Source: CAD feature listing. Evaluate the final solid. Frame: model axes, mm. Face numbers are marked on the shaded views. A direction names the side the tool comes from. Give positions to 0.01 mm unless a question says otherwise; leave off trailing zeros. Order: outer loops, then holes, each group sorted by start corner. A loop starts at its lowest first (then second) coordinate and runs counter-clockwise, first axis right, second up. Notation, with made-up numbers: M 35.5,42.5 L 63.5,42.5 A5 cw 63.5,50.5 Z; hole C -18,-4.5 d11. An arc over 180 degrees is marked long. Answer as a JSON object with one key per item and string values. Group by question number.
1. Material intervals for L1, parallel to Y at x = 13, z = 5.25; L2, parallel to X at y = 5, z = 1.7 (3 decimals); L3, parallel to Z at x = -3.5, y = 8.5, sorted ascending. Write a range as [from, to].
2. Set-up query: the marked faces 1, 2, 3 and 4. Return all of +Z, -Z, +X, -X, +Y, -Y with unobstructed straight access to the full face (end or side cutting, diameter ignored); none if empty.
3. Section query B-B (y = 0). Output: boundary loops of the cut face in (x, z) (3 decimals).
4. Pull-direction query (Y, two-part tool) for the marked faces 5, 6 and 7; classes: +Y half, -Y half, draft (parallel to the pull), parting line (faces both ways), or undercut.
5. Section query C-C (z = 4). Output: boundary loops of the cut face in (x, y), plus the area to 3 significant figures.
6. Pin query (flat end, axial travel): P1, Ø1.1, axis at x = 0.5, y = 1, coming from the -Z side; P2, Ø10, axis at x = 2.5, y = 8, coming from the -Z side; P3, Ø3, axis at x = 2, z = 4, coming from the +Y side. Return the tip coordinate at first contact, or that it passes through.
7. Section query A-A (x = -10.5). Output: boundary loops of the cut face in (y, z), plus the area to 3 significant figures.
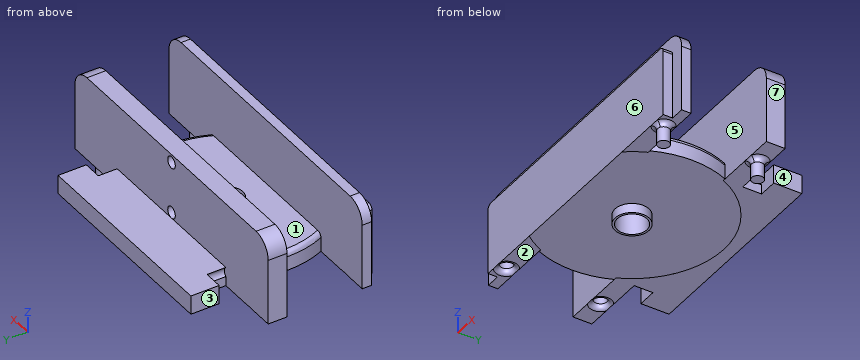
from build123d import *

# Parameters (mm, degrees)
BOSS_EXTRUDE1_DEPTH     = 2
SKETCH2_R               = 1.575
BOSS_EXTRUDE2_DEPTH     = 4
SKETCH3_R               = 1.8
BOSS_EXTRUDE3_DEPTH     = 1
SKETCH4_W               = 2
SKETCH4_H               = 17
BOSS_EXTRUDE4_DEPTH     = 0.001
SKETCH5_W               = 18
SKETCH5_H               = 2
BOSS_EXTRUDE5_DEPTH     = 0.001
SKETCH6_W               = 2.001
SKETCH6_H               = 2
BOSS_EXTRUDE6_DEPTH     = 5
BOSS_EXTRUDE7_DEPTH     = 0.001
CUT_EXTRUDE1_DEPTH      = 20.519323784
SKETCH9_W               = 2.937742252
SKETCH9_H               = 8
CUT_EXTRUDE2_DEPTH      = 0.001
CUT_EXTRUDE11_START     = -0.001
SKETCH21_R              = 9.75
SKETCH21_R_2            = 1.8
CUT_EXTRUDE11_DEPTH     = 0.001
SKETCH10_W              = 32
SKETCH10_H              = 2
BOSS_EXTRUDE8_DEPTH     = 7
FILLET1_R               = 0.5
SKETCH11_R              = 0.625
BOSS_EXTRUDE9_DEPTH     = 2
SKETCH14_W              = 2
SKETCH14_H              = 2
CUT_EXTRUDE5_DEPTH      = 22.401355237
SKETCH12_R              = 0.675
CUT_EXTRUDE3_DEPTH      = 2.5
CUT_EXTRUDE6_DEPTH      = 2
FILLET2_R               = 0.5
FILLET3_R               = 0.5
FILLET4_R               = 2
CUT_EXTRUDE7_DEPTH      = 26.019992106
CUT_EXTRUDE7_DEPTH_BACK = 1
SKETCH19_R              = 0.625
CUT_EXTRUDE9_DEPTH      = 2


with BuildPart() as part:
    # Sketch1 → Boss-Extrude1 (new body)
    with BuildSketch(Plane.XY):
        Polygon((-11, 6), (-11, 11), (11, 11), (11, 6), (11, -6), (-11, -6), align=None)
    extrude(amount=BOSS_EXTRUDE1_DEPTH)

    # Sketch3 → Boss-Extrude3 (add)
    with BuildSketch(Plane(origin=(0, 0, 0), x_dir=(-1, 0, 0), z_dir=(0, 0, -1))):
        with Locations(Location((0, 0, 0), (0, 0, 180))):
            Circle(SKETCH3_R)
    extrude(amount=BOSS_EXTRUDE3_DEPTH)

    # Sketch4 → Boss-Extrude4 (add)
    with BuildSketch(Plane(origin=(0, 0, 0), x_dir=(-1, 0, 0), z_dir=(0, 0, -1))):
        with Locations((10, 2.5)):
            Rectangle(SKETCH4_W, SKETCH4_H)
        with Locations((-10, 2.5)):
            Rectangle(SKETCH4_W, SKETCH4_H)
    extrude(amount=BOSS_EXTRUDE4_DEPTH)

    # Sketch5 → Boss-Extrude5 (add)
    with BuildSketch(Plane(origin=(0, 0, 0), x_dir=(-1, 0, 0), z_dir=(0, 0, -1))):
        with Locations((0, 10)):
            Rectangle(SKETCH5_W, SKETCH5_H)
    extrude(amount=BOSS_EXTRUDE5_DEPTH)

    # Sketch6 → Boss-Extrude6 (add)
    with BuildSketch(Plane(origin=(11, 0, 0), x_dir=(0, 0, -1), z_dir=(1, 0, 0))):
        with Locations((-0.9995, -5)):
            Rectangle(SKETCH6_W, SKETCH6_H)
        with Locations((-0.9995, 5)):
            Rectangle(SKETCH6_W, SKETCH6_H)
    boss_extrude6 = extrude(amount=BOSS_EXTRUDE6_DEPTH)

    # Mirror1: Boss-Extrude6 across plane
    add(boss_extrude6.mirror(Plane(origin=(0, 0, 0), x_dir=(0, 0, 1), z_dir=(1, 0, 0))))

    # Sketch7 → Boss-Extrude7 (add)
    with BuildSketch(Plane(origin=(0, 0, -0.001), x_dir=(-1, 0, 0), z_dir=(0, 0, -1))):
        with BuildLine():
            ThreePointArc((-6.708203932, -6), (-8.407551231, -3.211398808), (-9, 0))
            Line((-9, 0), (-9, -6))
            Line((-9, -6), (-6.708203932, -6))
        make_face()
        with BuildLine():
            Line((-9, 9), (-9, 0))
            ThreePointArc((-9, 0), (-6.363961031, 6.363961031), (0, 9))
            Line((0, 9), (-9, 9))
        make_face()
    boss_extrude7 = extrude(amount=-BOSS_EXTRUDE7_DEPTH)

    # Sketch8 → Cut-Extrude1 (cut, through all)
    with BuildSketch(Plane(origin=(0, 0, -0.001), x_dir=(-1, 0, 0), z_dir=(0, 0, -1))):
        with BuildLine():
            Line((-11, 4), (-9.16515139, 4))
            ThreePointArc((-9.16515139, 4), (-10, 0), (-9.16515139, -4))
            Line((-9.16515139, -4), (-11, -4))
            Line((-11, -4), (-11, 4))
        make_face()
    cut_extrude1 = extrude(amount=-CUT_EXTRUDE1_DEPTH, mode=Mode.SUBTRACT)

    # Sketch9 → Cut-Extrude2 (cut)
    with BuildSketch(Plane(origin=(0, 0, -0.001), x_dir=(-1, 0, 0), z_dir=(0, 0, -1))):
        with Locations((-9.531128874, 0)):
            Rectangle(SKETCH9_W, SKETCH9_H)
    cut_extrude2 = extrude(amount=-CUT_EXTRUDE2_DEPTH, mode=Mode.SUBTRACT)

    # Mirror2: Boss-Extrude7, Cut-Extrude1, Cut-Extrude2 across plane
    add(boss_extrude7.mirror(Plane(origin=(0, 0, 0), x_dir=(0, 0, 1), z_dir=(1, 0, 0))))
    add(cut_extrude1.mirror(Plane(origin=(0, 0, 0), x_dir=(0, 0, 1), z_dir=(1, 0, 0))), mode=Mode.SUBTRACT)
    add(cut_extrude2.mirror(Plane(origin=(0, 0, 0), x_dir=(0, 0, 1), z_dir=(1, 0, 0))), mode=Mode.SUBTRACT)

    # Sketch21 → Cut-Extrude11 (cut)
    with BuildSketch(Plane(origin=(0, 0, -0.001), x_dir=(-1, 0, 0), z_dir=(0, 0, -1)).offset(CUT_EXTRUDE11_START)):
        Circle(SKETCH21_R)
        with Locations(Location((0, 0, 0), (0, 0, 180))):
            Circle(SKETCH21_R_2, mode=Mode.SUBTRACT)
    extrude(amount=CUT_EXTRUDE11_DEPTH, mode=Mode.SUBTRACT)

    # Sketch10 → Boss-Extrude8 (add)
    with BuildSketch(Plane.XY.offset(2)):
        with Locations((0, -5)):
            Rectangle(SKETCH10_W, SKETCH10_H)
        with Locations((0, 5)):
            Rectangle(SKETCH10_W, SKETCH10_H)
    extrude(amount=BOSS_EXTRUDE8_DEPTH)

    # Fillet1
    fillet1_edges = [part.edges().sort_by_distance(p)[0] for p in [
        (10, 0, 2),
        (-10, 0, 2),
    ]]
    fillet(fillet1_edges, radius=FILLET1_R)

    # Sketch11 → Boss-Extrude9 (add)
    with BuildSketch(Plane(origin=(0, 0, -0.001), x_dir=(-1, 0, 0), z_dir=(0, 0, -1))):
        with Locations(Location((-13, -5, 0), (0, 0, 180))):
            Circle(SKETCH11_R)
    boss_extrude9 = extrude(amount=BOSS_EXTRUDE9_DEPTH)

    # Sketch14 → Cut-Extrude5 (cut, through all)
    with BuildSketch(Plane(origin=(0, 0, -0.001), x_dir=(-1, 0, 0), z_dir=(0, 0, -1))):
        with Locations((10, 7)):
            Rectangle(SKETCH14_W, SKETCH14_H)
        with Locations((-10, 7)):
            Rectangle(SKETCH14_W, SKETCH14_H)
    extrude(amount=-CUT_EXTRUDE5_DEPTH, mode=Mode.SUBTRACT)

    # Sketch12 → Cut-Extrude3 (cut)
    with BuildSketch(Plane(origin=(0, 0, -0.001), x_dir=(-1, 0, 0), z_dir=(0, 0, -1))):
        with Locations((13, -5)):
            Circle(SKETCH12_R)
    cut_extrude3 = extrude(amount=-CUT_EXTRUDE3_DEPTH, mode=Mode.SUBTRACT)

    # Sketch16 → Cut-Extrude6 (cut)
    with BuildSketch(Plane(origin=(0, 6, 0), x_dir=(1, 0, 0), z_dir=(0, 1, 0))):
        with BuildLine():
            Line((-9, -1), (-9, -2))
            ThreePointArc((-9, -2), (-8.75, -1.5), (-9, -1))
        make_face()
    cut_extrude6 = extrude(amount=CUT_EXTRUDE6_DEPTH, mode=Mode.SUBTRACT)

    # Mirror3: Boss-Extrude9, Cut-Extrude3 across plane
    add(boss_extrude9.mirror(Plane.ZX))
    add(cut_extrude3.mirror(Plane.ZX), mode=Mode.SUBTRACT)

    # Mirror4: Cut-Extrude6 across plane
    add(cut_extrude6.mirror(Plane(origin=(0, 0, 0), x_dir=(0, 0, 1), z_dir=(1, 0, 0))), mode=Mode.SUBTRACT)

    # Fillet2
    fillet2_edges = [part.edges().sort_by_distance(p)[0] for p in [
        (12.375, -5, -0.001),
        (12.375, 5, -0.001),
    ]]
    fillet(fillet2_edges, radius=FILLET2_R)

    # Fillet3
    # the kernel refuses this fillet: 0.5 mm, written as the material it takes off along each edge
    with BuildSketch(Plane(origin=(-13, -5, -0.001), x_dir=(-1, 0, 0), z_dir=(0, -1, 0))) as fillet3_piece_1:
        with BuildLine():
            CenterArc((0.675 + FILLET3_R, -FILLET3_R), FILLET3_R, 90, 90)
            Line((0.675, -FILLET3_R), (0.675, 0))
            Line((0.675, 0), (0.675 + FILLET3_R, 0))
        make_face()
    revolve(axis=Axis((-13, -5, -0.001), (0, 0, -1)), mode=Mode.SUBTRACT)
    with BuildSketch(Plane(origin=(-13, 5, -0.001), x_dir=(-1, 0, 0), z_dir=(0, 1, 0))) as fillet3_piece_2:
        with BuildLine():
            CenterArc((0.675 + FILLET3_R, FILLET3_R), FILLET3_R, 180, 90)
            Line((0.675, FILLET3_R), (0.675, 0))
            Line((0.675, 0), (0.675 + FILLET3_R, 0))
        make_face()
    revolve(axis=Axis((-13, 5, -0.001), (0, 0, 1)), mode=Mode.SUBTRACT)

    # Fillet4
    fillet4_edges = [part.edges().sort_by_distance(p)[0] for p in [
        (16, -5, 9),
        (-16, -5, 9),
        (-16, 5, 9),
        (16, 5, 9),
    ]]
    fillet(fillet4_edges, radius=FILLET4_R)

    # Sketch17 → Cut-Extrude7 (cut, two sides: drawn at the far end of the back side and taken through both)
    with BuildSketch(Plane.XZ.offset(6).offset(-CUT_EXTRUDE7_DEPTH_BACK)):
        with BuildLine():
            Line((-16, 7), (-16, -0.001))
            Line((-16, -0.001), (-14.5, -0.001))
            Line((-14.5, -0.001), (-14.5, 7))
            ThreePointArc((-14.5, 7), (-14.353553391, 7.353553391), (-14, 7.5))
            Line((-14, 7.5), (14, 7.5))
            ThreePointArc((14, 7.5), (14.353553391, 7.353553391), (14.5, 7))
            Line((14.5, 7), (14.5, -0.001))
            Line((14.5, -0.001), (16, -0.001))
            Line((16, -0.001), (16, 7))
            ThreePointArc((16, 7), (15.414213562, 8.414213562), (14, 9))
            Line((14, 9), (-14, 9))
            ThreePointArc((-14, 9), (-15.414213562, 8.414213562), (-16, 7))
        make_face()
    extrude(amount=CUT_EXTRUDE7_DEPTH + CUT_EXTRUDE7_DEPTH_BACK, mode=Mode.SUBTRACT)

    # Sketch19 → Cut-Extrude9 (cut)
    with BuildSketch(Plane(origin=(0, 6, 0), x_dir=(1, 0, 0), z_dir=(0, 1, 0))):
        with Locations(Location((0, -2.625, 0), (0, 0, 90))):
            Circle(SKETCH19_R)
        with Locations(Location((0, -8.125, 0), (0, 0, 270))):
            Circle(SKETCH19_R)
    extrude(amount=-CUT_EXTRUDE9_DEPTH, mode=Mode.SUBTRACT)


with BuildPart() as body_2:
    # Sketch2 → Boss-Extrude2 (new body)
    with BuildSketch(Plane(origin=(0, 0, 2), x_dir=(-1, 0, 0), z_dir=(0, 0, -1))):
        Circle(SKETCH2_R)
    extrude(amount=BOSS_EXTRUDE2_DEPTH)


with BuildPart() as part_1:
    add(part.part)

    # Combine2: cut body 2
    add(body_2.part, mode=Mode.SUBTRACT)


solid = part_1.part
Answer sheet:
{
 "1": {"L1": "[-6, -4], [4, 6]", "L2": "[-16, -13.675], [-12.325, 16]", "L3": "[0, 2]"},
 "2": {"face 1": "+Z, +X, -X", "face 2": "-Z, -X, +Y, -Y", "face 3": "+Z, -Z, -X, +Y", "face 4": "+Z, -Z, +X, +Y"},
 "3": {"outline": "M -10,0 L -1.8,0 L -1.8,-1 L -1.575,-1 L -1.575,2 L -9.5,2 A0.5 ccw -10,1.5 Z; M 1.575,-1 L 1.8,-1 L 1.8,0 L 10,0 L 10,1.5 A0.5 ccw 9.5,2 L 1.575,2 Z"},
 "4": {"face 5": "undercut", "face 6": "-Y half", "face 7": "draft"},
 "5": {"outline": "M -16,-5 L -14.5,-5 L -14.5,-6 L 14.5,-6 L 14.5,-5 L 16,-5 L 16,-4 L -16,-4 Z; M -16,4 L 16,4 L 16,6 L -16,6 Z", "area": "125 mm^2"},
 "6": {"P1": "z = -1", "P2": "z = 0", "P3": "y = 6"},
 "7": {"outline": "M -6,0 L -4,0 L -4,9 L -5,9 L -5,7.5 L -6,7.5 Z; M 4,0 L 6,0 L 6,9 L 4,9 Z; M 8,0 L 11,0 L 11,2 L 8,2 Z", "area": "40.5 mm^2"}
}
